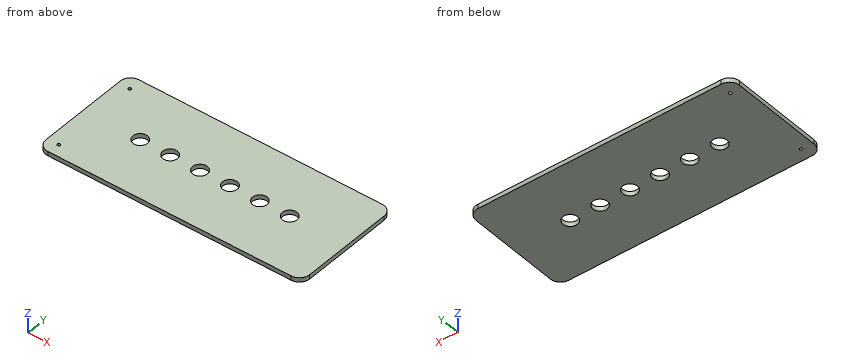
Autodesk Fusion 360 part; units mm, degrees
sketch "スケッチ1" plane through (0, 0, 0) normal (0, 0, 1) x (1, 0, 0)
  line L0 (3.5, 0) -> (86.5, 0)
  line L1 (90, 3.5) -> (90, 35)
  line L2 (86.5, 38.5) -> (3.5, 38.5)
  line L3 (0, 35) -> (0, 3.5)
  line L4 (0, 19.25) -> (90, 19.25)
  arc A0 (3.5, 38.5) -> (0, 35) centre (3.5, 35) ccw
  arc A1 (90, 35) -> (86.5, 38.5) centre (86.5, 35) ccw
  arc A2 (86.5, 0) -> (90, 3.5) centre (86.5, 3.5) ccw
  arc A3 (0, 3.5) -> (3.5, 0) centre (3.5, 3.5) ccw
  point P0 (90, 0)
  point P1 (0, 38.5)
  dimension "d1" = 90
  dimension "d2" = 38.5
  dimension "d3" = 3.5
extrude "押し出し1" add sketch "スケッチ1" along normal blind 1.5
sketch "スケッチ2" plane through (0, 0, 1.5) normal (0, 0, 1) x (-1, 0, 0)
  arc A0 (0, -3.5) -> (-3.5, 0) centre (-3.5, -3.5) ccw
  line L0 (-3.5, 0) -> (-86.5, 0)
  arc A1 (-86.5, 0) -> (-90, -3.5) centre (-86.5, -3.5) ccw
  line L1 (-90, -3.5) -> (-90, -35)
  arc A2 (-90, -35) -> (-86.5, -38.5) centre (-86.5, -35) ccw
  line L2 (-86.5, -38.5) -> (-3.5, -38.5)
  arc A3 (-3.5, -38.5) -> (0, -35) centre (-3.5, -35) ccw
  line L3 (0, -35) -> (0, -3.5)
  line L4 (-45, -38.5) -> (-45, 0)
  line L5 (0, -19.25) -> (-90, -19.25)
  line L6 (-45, -19.25) -> (-50.1, -19.25)
  line L7 (-50.1, -19.25) -> (-60.3, -19.25)
  line L8 (-60.3, -19.25) -> (-70.5, -19.25)
  point P0 (-50.1, -19.25)
  point P1 (-60.3, -19.25)
  point P2 (-70.5, -19.25)
  point P3 (-39.9, -19.25)
  point P4 (-29.7, -19.25)
  point P5 (-19.5, -19.25)
  dimension "d6" = 5.1
  dimension "d7" = 10.2
  dimension "d8" = 10.2
hole "穴1" at (19.5, 19.25, 1.5) at (29.7, 19.25, 1.5) at (39.9, 19.25, 1.5) at (50.1, 19.25, 1.5) at (60.3, 19.25, 1.5) at (70.5, 19.25, 1.5) direction (0, 0, -1) diameter 5 depth 1.5 tip angle 180
sketch "スケッチ3" plane through (0, 0, 1.5) normal (0, 0, 1) x (-1, 0, 0)
  circle A0 centre (-60.3, -19.25) radius 2.5
  circle A1 centre (-39.9, -19.25) radius 2.5
  circle A2 centre (-19.5, -19.25) radius 2.5
  circle A3 centre (-29.7, -19.25) radius 2.5
  circle A4 centre (-50.1, -19.25) radius 2.5
  circle A5 centre (-70.5, -19.25) radius 2.5
  arc A6 (0, -3.5) -> (-3.5, 0) centre (-3.5, -3.5) ccw
  line L0 (-3.5, 0) -> (-86.5, 0)
  arc A7 (-86.5, 0) -> (-90, -3.5) centre (-86.5, -3.5) ccw
  line L1 (-90, -3.5) -> (-90, -35)
  arc A8 (-90, -35) -> (-86.5, -38.5) centre (-86.5, -35) ccw
  line L2 (-86.5, -38.5) -> (-3.5, -38.5)
  arc A9 (-3.5, -38.5) -> (0, -35) centre (-3.5, -35) ccw
  line L3 (0, -35) -> (0, -3.5)
  line L4 (-4, -4) -> (-4, -34)
hole "穴2" at (4, 4, 1.5) at (4, 34, 1.5) direction (0, 0, -1) diameter 1 depth 1.5 tip angle 180
sketch "スケッチ5" plane through (0, 0, 0) normal (0, 0, 1) x (1, 0, 0)
sketch "スケッチ6" plane through (0, 0, 0) normal (0, 0, 1) x (1, 0, 0)
Design review of the part built by this model. Coordinates are the model's own, in mm. Coordinates: 2 decimals unless noted, no trailing zeros. Order: outer loops, then holes, each group sorted by start corner. A loop starts at its lowest first (then second) coordinate and runs counter-clockwise, first axis right, second up. Notation, with made-up numbers: (60.25, 0) -> (109.25, 0) arc R28 ccw to (109.25, 25) -> close; hole circle Ø10 at (76, 71). An arc over 180 degrees is marked (long way). One line per item, written item: value.
1) We need section C-C, the plane x = 31. Give the boundary of the cut face in (y, z), then the cut area to 3 significant figures.
Output values:
outline: (0, 0) -> (17.11, 0) -> (17.11, 1.5) -> (0, 1.5) -> close; (21.39, 0) -> (38.5, 0) -> (38.5, 1.5) -> (21.39, 1.5) -> close
area: 51.3 mm2
2) We need section B-B, the plane z = 0.3. Count the separate pieces of the cut face and the enclosed holes in it, then the cut area to 3 significant figures.
Output values:
separate pieces: 1
enclosed holes: 8
area: 3,340 mm2
3) To check wall thickness, follow probe 1 along Y at (x, z) = (4, 1.15); probe 2 along Y at (x, z) = (50.1, 1.1); probe 3 along Y at (x, z) = (21, 0.8). State the ranges of each line that lie inside material, in increasing order. Write a range as [from, to].
Output values:
probe 1: y = [0, 3.5], [4.5, 33.5], [34.5, 38.5]
probe 2: y = [0, 16.75], [21.75, 38.5]
probe 3: y = [0, 17.25], [21.25, 38.5]
4) We need section A-A, the plane x = 60.3. Give the boundary of the cut face in (y, z), then the cut area to 4 significant figures.
Output values:
outline: (0, 0) -> (16.75, 0) -> (16.75, 1.5) -> (0, 1.5) -> close; (21.75, 0) -> (38.5, 0) -> (38.5, 1.5) -> (21.75, 1.5) -> close
area: 50.25 mm2
5) Clearance check with flat-ended pins moving along their axes: P1, Ø3, axis at x = 60.3, y = 19.25, coming from the +Z side; P2, Ø8, axis at x = 70.5, y = 19.25, coming from the -Z side. State where each tip first meets the part, or that it passes through.
Output values:
P1: passes through
P2: stops at z = 0
